Can you work these out from the model? Positions are in its coordinate system, mm. A direction names the side the tool comes from. Coordinates: 2 decimals unless noted, no trailing zeros. Loops run counter-clockwise (first coordinate to the right, second up) from the corner with the lowest first, then second, coordinate; pieces in that order, holes last. Notation, with made-up numbers: (49.25, 35) -> (55.25, 35) arc R17 cw to (55.25, 44) -> close; hole circle Ø7 at (32.5, 10.25). An arc over 180 degrees is marked (long way). Put each result on its own line as item: value. Start each with the question number.
Item 1: Please list where these lines run through material, in increasing order: L1, parallel to Y at x = 0, z = -2.25; L2, parallel to Z at x = 0.15, y = -2.75; L3, parallel to Y at x = 0.3, z = 3.5. Write a range as from..to.
Item 2: We'd pull the mould along Y, two halves only. Please class faces 3 (the flat face through (0.35, 0, -2)), 4 (the cylindrical face through (0.005, -0.158, -4.422)), 5 (the cylindrical face through (0, 2.6, -1.77)): pulls with the +Y half, pulls with the -Y half, needs draft (parallel to the pull), parting line crosses it, or undercut.
Item 3: If we section it at A-A on z = 0.75: Please give me the cut outline in (x, y).
Item 4: For faces 1 (the flat face through (-0.35, 0, -2)), 2 (the cylindrical face through (0, -2.58, -1.8)), which set-ups out of +Z, -Z, +X, -X, +Y, -Y let a thin tool reach every point of the face, with its end or its side?
Item 5: If we section it at C-C on y = 0: Please give me the cut outline in (x, z) (3 decimals), plus the area to 3 significant figures.
```python
from build123d import *

# Parameters (mm, degrees)
RESSALTO_EXTRUS_O1_DEPTH = 0.7


with BuildPart() as part:
    # Esboço1 → Ressalto-extrusão1 (new body)
    with BuildSketch(Plane(origin=(0.35, 0, 0), x_dir=(0, 0, -1), z_dir=(1, 0, 0))):
        with BuildLine():
            Line((-1.104601172, -1.2525), (-3.423938468, -1.828316235))
            ThreePointArc((-3.423938468, -1.828316235), (-3.714684542, -2.08501745), (-3.671190238, -2.470422481))
            ThreePointArc((-3.671190238, -2.470422481), (4.425, 0), (-3.671190238, 2.470422481))
            ThreePointArc((-3.671190238, 2.470422481), (-3.714684542, 2.08501745), (-3.423938468, 1.828316235))
            Line((-3.423938468, 1.828316235), (-1.104601172, 1.2525))
            ThreePointArc((-1.104601172, 1.2525), (-0.590434162, 1.562141959), (0, 1.67))
            Line((0, 1.67), (0, 2.693254687))
            ThreePointArc((0, 2.693254687), (0.146851884, 3.012300306), (0.484714793, 3.108239019))
            ThreePointArc((0.484714793, 3.108239019), (1.788476887, 2.587942939), (2.736118813, 1.552337615))
            ThreePointArc((2.736118813, 1.552337615), (2.765828941, 1.202376345), (2.519309074, 0.952209327))
            Line((2.519309074, 0.952209327), (1.562141959, 0.590434162))
            ThreePointArc((1.562141959, 0.590434162), (1.67, 0), (1.562141959, -0.590434162))
            Line((1.562141959, -0.590434162), (2.519309074, -0.952209327))
            ThreePointArc((2.519309074, -0.952209327), (2.765828941, -1.202376345), (2.736118813, -1.552337615))
            ThreePointArc((2.736118813, -1.552337615), (1.788476887, -2.587942939), (0.484714793, -3.108239019))
            ThreePointArc((0.484714793, -3.108239019), (0.146851884, -3.012300306), (0, -2.693254687))
            Line((0, -2.693254687), (0, -1.67))
            ThreePointArc((0, -1.67), (-0.590434162, -1.562141959), (-1.104601172, -1.2525))
        make_face()
    extrude(amount=-RESSALTO_EXTRUS_O1_DEPTH)


solid = part.part
```
Solutions:
1. L1: -3.81..-2.2, -0.85..0.85, 2.2..3.81
1. L2: -3.47..-1.53, 0..3.47
1. L3: -2.71..-1.86, 1.86..2.71
2. face 3: needs draft
2. face 4: parting line crosses it
2. face 5: undercut
3. outline: (-0.35, -4.36) -> (0.35, -4.36) -> (0.35, -1.49) -> (-0.35, -1.49) -> close; (-0.35, 1.49) -> (0.35, 1.49) -> (0.35, 4.36) -> (-0.35, 4.36) -> close
4. face 1: +Z, -Z, -X, +Y, -Y
4. face 2: +X, -X
5. outline: (-0.35, -4.425) -> (0.35, -4.425) -> (0.35, -1.67) -> (-0.35, -1.67) -> close
5. area: 1.93 mm^2
